```python
from build123d import *

# Parameters (mm, degrees)
SCHIZZO1_R                   = 2
ESTRUSIONE_ESTRUSIONE1_DEPTH = 3


with BuildPart() as part:
    # Schizzo1 → Estrusione-Estrusione1 (new body)
    with BuildSketch(Plane.XY):
        with BuildLine():
            Line((0, 20), (0, 475))
            Line((0, 475), (154.5, 475))
            Line((154.5, 475), (154.5, 415))
            ThreePointArc((154.5, 415), (157.428932188, 407.928932188), (164.5, 405))
            Line((164.5, 405), (284.5, 405))
            ThreePointArc((284.5, 405), (291.571067812, 407.928932188), (294.5, 415))
            Line((294.5, 415), (294.5, 475))
            Line((294.5, 475), (449, 475))
            Line((449, 475), (449, 20))
            Line((449, 20), (429, 0))
            Line((429, 0), (20, 0))
            Line((20, 0), (0, 20))
        make_face()
        with Locations((144.5, 425)):
            Circle(SCHIZZO1_R, mode=Mode.SUBTRACT)
        with Locations((224.5, 385)):
            Circle(SCHIZZO1_R, mode=Mode.SUBTRACT)
        with Locations((73.921872489, 445)):
            Circle(SCHIZZO1_R, mode=Mode.SUBTRACT)
        with Locations((9, 223.826386399)):
            Circle(SCHIZZO1_R, mode=Mode.SUBTRACT)
        with Locations((440, 224.5)):
            Circle(SCHIZZO1_R, mode=Mode.SUBTRACT)
        with Locations(Location((73.921872489, 405, 0), (0, 0, 180))):
            Circle(SCHIZZO1_R, mode=Mode.SUBTRACT)
        with Locations((375.078127511, 405)):
            Circle(SCHIZZO1_R, mode=Mode.SUBTRACT)
        with Locations(Location((375.078127511, 445, 0), (0, 0, 180))):
            Circle(SCHIZZO1_R, mode=Mode.SUBTRACT)
        with Locations(Location((144.5, 465, 0), (0, 0, 180))):
            Circle(SCHIZZO1_R, mode=Mode.SUBTRACT)
        with Locations(Location((304.5, 425, 0), (0, 0, 180))):
            Circle(SCHIZZO1_R, mode=Mode.SUBTRACT)
        with Locations((304.5, 465)):
            Circle(SCHIZZO1_R, mode=Mode.SUBTRACT)
        with BuildLine():
            Line((344.715899345, 435), (405.440355678, 435))
            ThreePointArc((405.440355678, 435), (415.440355678, 425), (405.440355678, 415))
            Line((405.440355678, 415), (344.715899345, 415))
            ThreePointArc((344.715899345, 415), (334.715899345, 425), (344.715899345, 435))
        make_face(mode=Mode.SUBTRACT)
        with BuildLine():
            Line((104.284100655, 435), (43.559644322, 435))
            ThreePointArc((43.559644322, 435), (33.559644322, 425), (43.559644322, 415))
            Line((43.559644322, 415), (104.284100655, 415))
            ThreePointArc((104.284100655, 415), (114.284100655, 425), (104.284100655, 435))
        make_face(mode=Mode.SUBTRACT)
        with BuildLine():
            Line((222.25, 15), (222.25, 25))
            ThreePointArc((222.25, 25), (224.5, 27.25), (226.75, 25))
            Line((226.75, 25), (226.75, 15))
            ThreePointArc((226.75, 15), (224.5, 12.75), (222.25, 15))
        make_face(mode=Mode.SUBTRACT)
    extrude(amount=ESTRUSIONE_ESTRUSIONE1_DEPTH)


solid = part.part
```
Design review of the part built by this model. Coordinates are the model's own, in mm. A direction names the side the tool comes from. Coordinates: 2 decimals unless noted, no trailing zeros. One line per item, written item: value. Start each with the question number.
Q1. Take a section at A-A, the plane z = 1.3. Give the number of separate pieces and of enclosed holes in the cut face, then the cut area to 3 significant figures.
Q2. Insertion check: pin 1 Ø0.9 at (x, z) = (61, 1) entering from -Y; pin 2 Ø0.9 at (y, z) = (18, 2) entering from -X. Each pin has a flat end and moves straight along its axis. Give the tip position at first contact, or say it passes through.
Q3. Mouldability with a two-part tool opening along X and no side actions: class faces 4 (the flat face through (228, 241, 0)), 5 (the flat face through (10, 10, 1)), 6 (the cylindrical face through (33.562, 425.22, 1.479)), 7 (the cylindrical face through (415.438, 425.22, 1.479)) as pulls with the +X half, pulls with the -X half, needs draft (parallel to the pull), parting line crosses it, or undercut.
Q4. Tool access review of faces 1 (the cylindrical face through (334.72, 424.78, 1.48)), 2 (the flat face through (439, 10, 1)), 3 (the cylindrical face through (291.49, 407.85, 1.48)): name each direction out of +Z, -Z, +X, -X, +Y, -Y from which nothing blocks a thin tool from reaching the whole face with its end or side.
Q5. For probe 1 along X at (y, z) = (425, 1.4); probe 2 along Y at (x, z) = (224.5, 2.4); probe 3 along X at (y, z) = (445, 1.6), list the stretches that pass through material, from the lowest coordinate up.
Values follow:
1. separate pieces: 1
1. enclosed holes: 14
1. area: 200,000 mm2
2. pin 1: stops at y = 0
2. pin 2: stops at x = 1.55
3. face 4: needs draft
3. face 5: pulls with the -X half
3. face 6: undercut
3. face 7: undercut
4. face 1: +Z, -Z
4. face 2: +Z, -Z, +X, -Y
4. face 3: +Z, -Z, +Y
5. probe 1: x = 0 to 33.56, 114.28 to 142.5, 146.5 to 154.5, 294.5 to 302.5, 306.5 to 334.72, 415.44 to 449
5. probe 2: y = 0 to 12.75, 27.25 to 383, 387 to 405
5. probe 3: x = 0 to 71.92, 75.92 to 154.5, 294.5 to 373.08, 377.08 to 449
